Geometry: final body of the model. Coordinates: model frame, mm. A direction names the side the tool comes from. Round coordinates to 2 decimals unless told otherwise and drop trailing zeros. Write each loop counter-clockwise with the first axis right and the second up, starting at its lowest first coordinate (ties: lowest second). Pieces come first, ordered by that corner, then holes. Notation, with made-up numbers: (43, 85) -> (80, 85) arc R26 cw to (80, 106) -> close; hole circle Ø9 at (-3.5, 19.25). An arc over 180 degrees is marked (long way). One line per item, written item: value. Start each with the question number.
from build123d import *

# Parameters (mm, degrees)
F0_R     = 30
F0_R_2   = 4
F1_DEPTH = 300
F2_R     = 10
F2_R_2   = 4
F3_DEPTH = 5
F4_R     = 10
F4_R_2   = 4
F5_DEPTH = 5


with BuildPart() as f1:
    # F0 (on Front) → F1 (new body)
    with BuildSketch(Plane.XZ):
        Circle(F0_R)
        Circle(F0_R_2, mode=Mode.SUBTRACT)
    extrude(amount=F1_DEPTH)

    # F2 (on face) → F3 (join)
    with BuildSketch(Plane.XZ.offset(300)):
        Circle(F2_R)
        Circle(F2_R_2, mode=Mode.SUBTRACT)
    extrude(amount=F3_DEPTH)

    # F4 (on face) → F5 (join)
    with BuildSketch(Plane(origin=(0, 0, 0), x_dir=(-1, 0, 0), z_dir=(0, 1, 0))):
        Circle(F4_R)
        Circle(F4_R_2, mode=Mode.SUBTRACT)
    extrude(amount=F5_DEPTH)


solid = f1.part
(1) Section query B-B (x = 0). Output: boundary loops of the cut face in (y, z), and give its area (3 significant figures).
(2) Set-up query: faces 1 (the face through (-2.17, -302.46, -9.76)), 2 (the face through (-29.97, -147.9, 1.32)), 3 (the face through (2.17, 2.46, -9.76)). Return all of +Z, -Z, +X, -X, +Y, -Y with unobstructed straight access to the full face (end or side cutting, diameter ignored); none if empty.
(3) Section query A-A (z = 0). Output: boundary loops of the cut face in (x, y).
(4) Section query C-C (y = -133.5). Output: boundary loops of the cut face in (x, z).
(5) Line query: probe 1 along Z at (x, y) = (0, 1); probe 2 along Z at (x, y) = (0, -119); probe 3 along Y at (x, z) = (8.5, -17). Output: solid intervals per line, ascending.
(6) Pin query (flat end, axial travel): pin 1 (3 mm diameter, centred on y = -155, z = 11, fed in from +X); pin 2 (1 mm diameter, centred on y = -168, z = -2, fed in from -X); pin 3 (6 mm diameter, centred on y = -65.5, z = 20, fed in from +X). Return the tip coordinate at first contact, or that it passes through.
(7) Section query D-D (x = -21.5). Output: boundary loops of the cut face in (y, z), and give its area (3 significant figures).
Results list:
1. outline: (-305, -10) -> (-300, -10) -> (-300, -30) -> (0, -30) -> (0, -10) -> (5, -10) -> (5, -4) -> (-305, -4) -> close; (-305, 4) -> (5, 4) -> (5, 10) -> (0, 10) -> (0, 30) -> (-300, 30) -> (-300, 10) -> (-305, 10) -> close
1. area: 15,700 mm^2
2. face 1: -Y
2. face 2: +Y, -Y
2. face 3: +Y
3. outline: (-30, -300) -> (-10, -300) -> (-10, -305) -> (-4, -305) -> (-4, 5) -> (-10, 5) -> (-10, 0) -> (-30, 0) -> close; (4, -305) -> (10, -305) -> (10, -300) -> (30, -300) -> (30, 0) -> (10, 0) -> (10, 5) -> (4, 5) -> close
4. outline: circle Ø60 at (0, 0); hole circle Ø8 at (0, 0)
5. probe 1: z = -10 to -4, 4 to 10
5. probe 2: z = -30 to -4, 4 to 30
5. probe 3: y = -300 to 0
6. pin 1: stops at x = 28.46
6. pin 2: stops at x = -29.96
6. pin 3: stops at x = 24.72
7. outline: (-300, -20.92) -> (0, -20.92) -> (0, 20.92) -> (-300, 20.92) -> close
7. area: 12,600 mm^2
